Autodesk Inventor part; units mm, degrees
ref_plane "YZ Plane" through (0, 0, 0) normal (1, 0, 0) x (0, 1, 0)
ref_plane "XZ Plane" through (0, 0, 0) normal (0, 1, 0) x (-1, 0, 0)
ref_plane "XY Plane" through (0, 0, 0) normal (0, 0, 1) x (1, 0, 0)
sketch "Sketch1" plane through (0, 0, 0) normal (0, 1, 0) x (-1, 0, 0)
  line L0 (-9.33, 18.36) -> (9.33, 18.36)
  line L1 (9.33, 18.36) -> (9.33, -18.36)
  line L2 (9.33, -18.36) -> (-9.33, -18.36)
  line L3 (-9.33, -18.36) -> (-9.33, 18.36)
  line L4 (9.33, 18.36) -> (-9.33, -18.36) construction
  point P0 (0, 0)
extrude "Extrusion1" add sketch "Sketch1" along normal blind 21
fillet "Fillet1" radius 5 2 edges at (0, 21, 18.36) (0, 0, 18.36)
sketch "Sketch2" plane through (9.33, 0, -18.36) normal (0, 0, -1) x (-1, 0, 0)
  circle A0 centre (9.33, 10.5) radius 10.5
  point P0 (9.33, 0)
extrude "Extrusion2" add sketch "Sketch2" along normal blind 10.7
sketch "Sketch3" plane through (9.33, 0, -18.36) normal (0, 0, 1) x (1, 0, 0)
  line L0 (0, 5.6832) -> (0, 15.3168)
  arc A0 (0, 5.6832) -> (0, 15.3168) centre (-9.33, 10.5) ccw
  line L1 (-18.66, 5.6832) -> (-18.66, 15.3168)
  arc A1 (-18.66, 15.3168) -> (-18.66, 5.6832) centre (-9.33, 10.5) ccw
  point P0 (-9.33, 0)
extrude "Extrusion3" cut sketch "Sketch3" against normal blind 10.7
sketch "Sketch4" plane through (9.33, 0, 13.36) normal (1, 0, 0) x (0, 0, -1)
  line L0 (36.17, 13) -> (38.67, 13)
  line L1 (38.67, 13) -> (38.67, 8)
  line L2 (38.67, 8) -> (36.17, 8)
  line L3 (36.17, 8) -> (36.17, 13)
  point P0 (13.36, 0)
extrude "Extrusion4" add sketch "Sketch4" along normal blind 3
mirror "Mirror1" about plane through (0, 0, 0) normal (1, 0, 0) of "Extrusion4"
sketch "Sketch5" plane through (9.33, 0, -29.06) normal (0, 0, -1) x (-1, 0, 0)
  arc A0 (18.66, 15.3168) -> (0, 15.3168) centre (9.33, 10.5) ccw
  line L0 (0.83, 10.5) -> (0.83, 14.7426)
  line L1 (0.83, 10.5) -> (0.83, 6.2574)
  line L2 (9.33, 10.5) -> (9.33, 11.5651)
  line L3 (17.83, 10.5) -> (17.83, 14.7426)
  line L4 (17.83, 10.5) -> (17.83, 6.2574)
  arc A1 (17.83, 14.7426) -> (0.83, 14.7426) centre (9.33, 10.5) ccw
  arc A2 (0.83, 6.2574) -> (17.83, 6.2574) centre (9.33, 10.5) ccw
  point P0 (9.33, 0)
  point P1 (0.83, 15.6468)
  point P2 (0.83, 5.1568)
  point P3 (17.83, 15.6468)
  point P4 (17.83, 5.1568)
extrude "Extrusion5" add sketch "Sketch5" along normal blind 12.74
fillet "Fillet2" radius 1 2 edges at (0, 20, -41.8) (0, 1, -41.8)
sketch "Sketch6" plane through (9.33, 0, -41.8) normal (0, 0, -1) x (-1, 0, 0)
  arc A0 (17.83, 10.5) -> (0.83, 10.5) centre (9.33, 10.5) ccw
  circle A1 centre (9.33, 10.5) radius 4.5
  point P0 (9.33, 0)
  dimension "d20" = 9
extrude "Extrusion6" add sketch "Sketch6" along normal blind 2.5
fillet "Fillet3" radius 0.5 1 edges at (4.5, 10.5, -44.3)
sketch "Sketch7" plane through (0, 10.5, -44.3) normal (0, 0, -1) x (-1, 0, 0)
  circle A0 centre (0, 0) radius 4
  circle A1 centre (0, 0) radius 4.5
  circle A2 centre (0, 0) radius 4
  line L0 (-3.0711, 4.7099) -> (3.07, 4.7099)
  line L1 (3.07, 4.7099) -> (3.07, 3.2901)
  line L2 (3.07, 3.2901) -> (-3.0711, 3.2901)
  line L3 (-3.0711, 3.2901) -> (-3.0711, 4.7099)
  line L4 (-3.0711, 4.7099) -> (3.07, 3.2901) construction
  line L5 (3.07, 4.7099) -> (-3.0711, 3.2901) construction
  point P0 (0, -10.5)
  point P1 (-0.0005, 4)
extrude "Extrusion7" cut sketch "Sketch7" against normal blind 2.5 contours L2 A0 | A0 L2 A1 | A1 L3 L0 L1 picked at (0.4734, 3.4399) picked at (1.9981, 3.6326)
sketch "Sketch8" plane through (9.33, 0, -44.3) normal (0, 0, -1) x (-1, 0, 0)
  arc A0 (7.0551, 13.7901) -> (11.6049, 13.7901) centre (9.33, 10.5) ccw
  circle A1 centre (9.33, 10.5) radius 0.5
  point P0 (9.33, 0)
  dimension "d26" = 1
extrude "Extrusion8" add sketch "Sketch8" along normal blind 0.5
sketch "Sketch9" plane through (-9.33, 5, 18.36) normal (0, 0, 1) x (1, 0, 0)
  line L0 (7.83, 8) -> (10.83, 8)
  line L1 (10.83, 8) -> (10.83, 3)
  line L2 (10.83, 3) -> (7.83, 3)
  line L3 (7.83, 3) -> (7.83, 8)
  line L4 (7.83, 8) -> (10.83, 3) construction
  line L5 (10.83, 8) -> (7.83, 3) construction
  point P0 (9.33, -5)
  point P1 (9.33, 5.5)
  dimension "d29" = 3
  dimension "d30" = 5
extrude "Extrusion9" add sketch "Sketch9" along normal blind 5
sketch "Sketch10" plane through (1.5, 8, 18.36) normal (1, 0, 0) x (0, 0, -1)
  circle A0 centre (-2.5, 2.5) radius 1.5
  point P0 (18.36, -8)
  dimension "d33" = 3
extrude "Extrusion10" cut sketch "Sketch10" against normal blind 5
fillet "Fillet4" radius 0.5 4 edges at (1.5, 10.5, 18.36) (0, 13, 18.36) (-1.5, 10.5, 18.36) (0, 8, 18.36)
sketch "Sketch11" plane through (9.33, 0, 13.36) normal (1, 0, 0) x (0, 0, -1)
  circle A0 centre (4.89, 10.5) radius 1.25
  point P0 (13.36, 0)
extrude "Extrusion11" add sketch "Sketch11" along normal blind 5
mirror "Mirror3" about plane through (0, 0, 0) normal (1, 0, 0) of "Extrusion11"
properties part number "motor_dc"
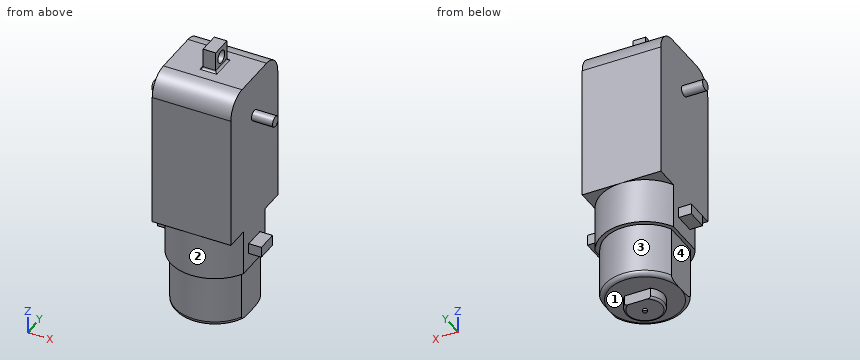
Here's how the part is built. I have some questions about the finished solid (model axes, mm). Face numbers are marked on the shaded views. A direction names the side the tool comes from. Coordinates: 2 decimals unless noted, no trailing zeros. Order: outer loops, then holes, each group sorted by start corner. A loop starts at its lowest first (then second) coordinate and runs counter-clockwise, first axis right, second up. Notation, with made-up numbers: M -4.75,-9 L 0.25,-9 A32 ccw 0.25,29 Z; hole C -23.75,-36.5 d8. An arc over 180 degrees is marked long. Answer as a JSON object with one key per item and string values. Group by question number.
(1) Suppose I cut it at C-C, the plane z = -12.5. Please give me the cut outline in (x, y), then the cut area to 3 significant figures.
(2) Suppose I cut it at A-A, the plane z = 20.86. Please give me the cut outline in (x, y), then the cut area to 3 significant figures.
(3) For pin 1 (4 mm diameter, centred on y = 12.5, z = -31.5, fed in from -X); pin 2 (5 mm diameter, centred on y = 17, z = 6, fed in from -X); pin 3 (3 mm diameter, centred on y = 13, z = 0.5, fed in from +X); pin 4 (5 mm diameter, centred on x = -4, z = 11, fed in from -Y), each with a flat end and sliding along its axis, tell me the tip position at first contact or that it passes through.
(4) Which directions (+Z, -Z, +X, -X, +Y, -Y) give clear straight access to the entire face, cutting with the end or side of a thin tool? Please do the marked faces 1, 2, 3 and 4.
(5) Suppose I cut it at B-B, the plane z = 8.47. Please give me the cut outline in (x, y).
(6) I need wall thicknesses on probe 1 along Y at (x, z) = (0.95, 20.86); probe 2 along X at (y, z) = (14.75, -28); probe 3 along Z at (x, y) = (1, 9.5). Which ranges of each line are inside material? Lowest first, please.
(7) Suppose I cut it at D-D, the plane z = -31. Please give me the cut outline in (x, y), then the cut area to 3 significant figures.
Values found:
{
 "1": {"outline": "M -9.33,0 L 9.33,0 L 9.33,21 L -9.33,21 Z", "area": "392 mm^2"},
 "2": {"outline": "M -1.5,8 L 1.5,8 L 1.5,9 L -1.5,9 Z; M -1.5,12 L 1.5,12 L 1.5,13 L -1.5,13 Z", "area": "6.00 mm^2"},
 "3": {"pin 1": "stops at x = -8.5", "pin 2": "stops at x = -9.33", "pin 3": "stops at x = 9.33", "pin 4": "stops at y = 0"},
 "4": {"face 1": "-Z", "face 2": "-Z, -Y", "face 3": "-Z, +Y", "face 4": "-Z, -X, +Y, -Y"},
 "5": {"outline": "M -14.33,9.25 L -9.33,9.25 L -9.33,0 L 9.33,0 L 9.33,9.25 L 14.33,9.25 L 14.33,11.75 L 9.33,11.75 L 9.33,21 L -9.33,21 L -9.33,11.75 L -14.33,11.75 Z"},
 "6": {"probe 1": "y = 8 to 9, 12 to 13", "probe 2": "x = -9.33 to 9.33", "probe 3": "z = -44.3 to 19.74, 21.98 to 23.36"},
 "7": {"outline": "M -8.5,6.26 A9.5 ccw 8.5,6.26 L 8.5,14.74 A9.5 ccw -8.5,14.74 Z", "area": "272 mm^2"}
}
